from build123d import *

# Parameters (mm, degrees)
F_10_32_TAPPED_HOLE1_D     = 4.0386
F_10_32_TAPPED_HOLE1_DEPTH = 50.8
F_10_32_TAPPED_HOLE1_TIP   = 1.213317848
CHAMFER1_SIZE              = 1.27


with BuildPart() as part:
    # Sketch1 → Revolve1 (revolve)
    with BuildSketch(Plane(origin=(0, 0, 0), x_dir=(0, 0, -1), z_dir=(1, 0, 0))):
        Polygon((0, 9.525), (101.6, 22.7076), (101.6, 31.75), (0, 31.75), align=None)
    revolve(axis=Axis((0, 0, 60.933225134), (0, 0, -1)))

    # #10-32 Tapped Hole1
    with Locations(Plane.XY):
        with Locations((0, 22.86), (22.86, 0), (0, -22.86), (-22.86, 0), (0, 0)):
            Hole(F_10_32_TAPPED_HOLE1_D / 2, depth=F_10_32_TAPPED_HOLE1_DEPTH)
            with Locations((0, 0, -(F_10_32_TAPPED_HOLE1_DEPTH + F_10_32_TAPPED_HOLE1_TIP / 2))):  # 118° drill point
                Cone(0, F_10_32_TAPPED_HOLE1_D / 2, F_10_32_TAPPED_HOLE1_TIP, mode=Mode.SUBTRACT)

    # Chamfer1
    chamfer1_edges = [part.edges().sort_by_distance(p)[0] for p in [
        (0, -31.75, 0),
    ]]
    chamfer(chamfer1_edges, length=CHAMFER1_SIZE)


solid = part.part
CAD build for the part. Positions are in the model's coordinates, mm. A direction names the side the tool comes from. Give positions to 0.01 mm unless a question says otherwise; leave off trailing zeros. Write each loop counter-clockwise with the first axis right and the second up, starting at its lowest first coordinate (ties: lowest second). Pieces come first, ordered by that corner, then holes. Notation, with made-up numbers: M -12.5,-37 L 27.5,-37 A34 cw 27.5,-7 Z; hole C 34.5,-1.75 d10. An arc over 180 degrees is marked long. Put each result on its own line as item: value. Start each with the question number.
(1) Flat gauge pins, fed straight in: pin 1 Ø4 at (x, y) = (8.5, 12.5) entering from +Z; pin 2 Ø12 at (y, z) = (-12.5, -21) entering from +X; pin 3 Ø1 at (y, z) = (13, -38) entering from +X; pin 4 Ø3.5 at (x, y) = (22.86, 0) entering from +Z. Where does each tip first touch, or does it go through?
(2) Band-saw the part on B-B, the plane z = -65. Write the cut outline in (x, y), and give its area (3 significant figures).
(3) Which spindle directions (+Z, -Z, +X, -X, +Y, -Y) get a long thin tool onto all of the face, cutting with end or side? Do faces 1 (the face through (24.877, 0.089, -25.756)), 2 (the face through (4.87, 15.46, -51.51)). Say none if no direction does.
(4) Band-saw the part on A-A, the plane z = -92.5. Write the cut outline in (x, y), and give its area (3 significant figures).
(5) Probe L1, parallel to X at y = 1, z = -36; L2, parallel to X at y = 0, z = -16; L3, parallel to X at y = 5, z = -58. List the from-to ranges inside material, lowest first.
(6) Mould opens along X. For faces 3 (the face through (-30.995, -6.883, -50.733)), 4 (the face through (7, -7, 0)), 5 (the face through (0.44, 20.89, -25.76)) say: +X half, -X half, draft (parallel to the pull), parting line (faces both ways), or undercut.
Response values:
1. pin 1: stops at z = 0
1. pin 2: stops at x = 31.08
1. pin 3: stops at x = 29.19
1. pin 4: stops at z = -50.96
2. outline: C 0,0 d63.5; hole C 0,0 d35.92
2. area: 2,150 mm2
3. face 1: +Z
3. face 2: -Z
4. outline: C 0,0 d63.5; hole C 0,0 d43.05
4. area: 1,710 mm2
5. L1: x = -31.73 to -24.61, -21.11 to -14.16, 14.16 to 21.11, 24.61 to 31.73
5. L2: x = -31.75 to -24.88, -20.84 to -11.6, 11.6 to 20.84, 24.88 to 31.75
5. L3: x = -31.35 to -16.3, 16.3 to 31.35
6. face 3: parting line
6. face 4: draft
6. face 5: undercut
